```python
from build123d import *

# Parameters (mm, degrees)
SKETCH_1_R          = 3.5
EXTRUDE_1_DEPTH     = 4
CUT_EXTRUDE_1_DEPTH = 2
SKETCH_3_R          = 2
EXTRUDE_2_DEPTH     = 18


with BuildPart() as part:
    # 草图1 → 凸台-拉伸1 (new body)
    with BuildSketch(Plane(origin=(0, 0, 0), x_dir=(0, 0, -1), z_dir=(1, 0, 0))):
        Circle(SKETCH_1_R)
    extrude(amount=EXTRUDE_1_DEPTH)

    # 草图2 → 切除-拉伸1 (cut)
    with BuildSketch(Plane.ZY):
        Polygon((1.525, -0.880459161), (1.525, 0.880459161), (0, 1.760918321), (-1.525, 0.880459161), (-1.525, -0.880459161), (0, -1.760918321), align=None)
    extrude(amount=-CUT_EXTRUDE_1_DEPTH, mode=Mode.SUBTRACT)

    # 草图3 → 凸台-拉伸2 (add)
    with BuildSketch(Plane(origin=(4, 0, 0), x_dir=(0, 0, -1), z_dir=(1, 0, 0))):
        Circle(SKETCH_3_R)
    extrude(amount=EXTRUDE_2_DEPTH)


solid = part.part
```
The listing builds one solid part. Answer for the finished solid, in the listing's coordinates (mm). A direction names the side the tool comes from. Coordinates: 2 decimals unless noted, no trailing zeros. Write each loop counter-clockwise with the first axis right and the second up, starting at its lowest first coordinate (ties: lowest second). Pieces come first, ordered by that corner, then holes.
Q1. Section A-A, the plane y = 0 is taken. Write down the section's boundary in (x, z) (3 decimals), then the cut area to 3 significant figures.
Returned:
outline: (0, -3.5) - (4, -3.5) - (4, -2) - (22, -2) - (22, 2) - (4, 2) - (4, 3.5) - (0, 3.5) - (0, 1.525) - (2, 1.525) - (2, -1.525) - (0, -1.525) - close
area: 93.9 mm2
Q2. Section D-D, the plane y = 2.5 is taken. Write down the section's boundary in (x, z), then the cut area to 3 significant figures.
Returned:
outline: (0, -2.45) - (4, -2.45) - (4, 2.45) - (0, 2.45) - close
area: 19.6 mm2
Q3. Given P1, Ø1, axis at x = 9.5, y = 1.5, coming from the +Z side; P2, Ø2, axis at x = 11.5, y = -2, coming from the -Z side; P3, Ø1, axis at x = 2.5, z = -2.5, coming from the +Y side, each flat-ended and moving along its own axis, determine where each tip first touches the part or whether it passes through.
Returned:
P1: stops at z = 1.73
P2: stops at z = -1.73
P3: stops at y = 2.87
Q4. The mould has two halves that part along Y. Classify faces 1 (the cylindrical face through (13, -2, 0)), 2 (the flat face through (4, -2, -2)), 3 (the flat face through (2, 0, 0)), 4 (the flat face through (1, 1.3, -0.8)): released by +Y, released by -Y, zero draft, split by the parting line, or undercut.
Returned:
face 1: split by the parting line
face 2: zero draft
face 3: undercut
face 4: undercut
Q5. Section C-C, the plane z = -0.5 is taken. Write down the section's boundary in (x, y), then the cut area to 3 significant figures.
Returned:
outline: (0, -3.46) - (4, -3.46) - (4, -1.94) - (22, -1.94) - (22, 1.94) - (4, 1.94) - (4, 3.46) - (0, 3.46) - (0, 1.47) - (2, 1.47) - (2, -1.47) - (0, -1.47) - close
area: 91.5 mm2
Q6. Find the intervals of material crossed by line 1 along X through (y, z) = (3, -1); line 2 along X through (y, z) = (0, -0.5); line 3 along Y through (x, z) = (1.5, 0.75), in increasing order.
Returned:
line 1: x = 0 to 4
line 2: x = 2 to 22
line 3: y = -3.42 to -1.33, 1.33 to 3.42
Q7. Section B-B, the plane x = 18.5 is taken. Write down the section's boundary in (y, z).
Returned:
outline: circle Ø4 at (0, 0)
Q8. Which of the six approach directions +Z, -Z, +X, -X, +Y, -Y give full straight-line access (tool end or side, diameter ignored) to faces 5 (the flat face through (0, 0, 2)), 6 (the flat face through (1, -1.3, -0.8))?
Returned:
face 5: +Z, -Z, -X, +Y, -Y
face 6: -X
